Here's how the part is built. I have some questions about the finished solid (model axes, mm). Face numbers are marked on the shaded views. A direction names the side the tool comes from. Round coordinates to 2 decimals unless told otherwise and drop trailing zeros. Write each loop counter-clockwise with the first axis right and the second up, starting at its lowest first coordinate (ties: lowest second). Pieces come first, ordered by that corner, then holes. Notation, with made-up numbers: (2, 39.25) - (27, 39.25) arc R17 cw to (27, 45.25) - close; hole circle Ø2 at (-24, 73.25). An arc over 180 degrees is marked (long way). Use one line per item in the form item = value. Start each with the question number.
1. If I drill on line 1 along Z through (x, y) = (546.45, 0); line 2 along X through (y, z) = (2.25, -6.5); line 3 along Y through (x, z) = (547.5, -6.25), over which ranges is the centre line in solid material (lowest first)?
2. I want a section at B-B, the plane z = 0. State how many separate pieces and enclosed holes the cut face has, plus the area to 3 significant figures.
3. I want a section at A-A, the plane y = 0. List the corners of the cut face in (x, z) for me, plus the area to 3 significant figures.
4. Will these pins go through, and if not, where does the flat tip stop? pin 1 (8 mm diameter, centred on y = 0, z = 0, fed in from -X); pin 2 (6 mm diameter, centred on x = 550, z = 0.5, fed in from +Y); pin 3 (1.5 mm diameter, centred on x = 552.5, z = -5.5, fed in from -Y); pin 4 (3.5 mm diameter, centred on x = 557.15, z = 0, fed in from -Y).
5. I want a section at C-C, the plane z = 8. List the corners of the cut face in (x, y) for me, plus the area to 3 significant figures.
6. Which directions (+Z, -Z, +X, -X, +Y, -Y) give clear straight access to the entire face, cutting with the end or side of a thin tool? Please do the marked faces 4 and 5.
7. I want a section at D-D, the plane y = -6. List the corners of the cut face in (x, z) for me, plus the area to 3 significant figures.
8. We'd pull the mould along Y, two halves only. Please class the marked faces 1, 2 and 3: +Y half, -Y half, draft (parallel to the pull), parting line (faces both ways), or undercut.
```python
from build123d import *

# Parameters (mm, degrees)
CUT_EXTRUDE1_DEPTH      = 561.867355885
CUT_EXTRUDE1_DEPTH_BACK = 561.867355885
SKETCH3_R               = 1.5
SKETCH13_R              = 1
CUT_EXTRUDE2_DEPTH      = 20.974512648


with BuildPart() as part:
    # Sketch2 → Revolve1 (revolve)
    with BuildSketch(Plane.XY, mode=Mode.PRIVATE) as revolve1_sk:
        Polygon((560.650925037, 5), (560.650925037, 7.5), (552.150925037, 7.5), (552.150925037, 6.5), (548.150925037, 6.5), (548.150925037, 7.5), (548.150925037, 11.016604582), (545.650925037, 11.016604582), (545.650925037, 5), align=None)
    revolve(revolve1_sk.sketch.rotate(Axis((542.916757592, 0, 0), (1, 0, 0)), 180), axis=Axis((542.916757592, 0, 0), (1, 0, 0)))

    # Sketch3 → Cut-Extrude1 (cut, two sides: drawn at the far end of the back side and taken through both)
    with BuildSketch(Plane(origin=(0, 0, 0), x_dir=(1, 0, 0), z_dir=(0, 1, 0)).offset(-CUT_EXTRUDE1_DEPTH_BACK)):
        with Locations(Location((557.150925037, 0, 0), (0, 0, 270))):
            Circle(SKETCH3_R)
    extrude(amount=CUT_EXTRUDE1_DEPTH + CUT_EXTRUDE1_DEPTH_BACK, mode=Mode.SUBTRACT)

    # Sketch13 → Cut-Extrude2 (cut, through all)
    with BuildSketch(Plane(origin=(548.150925037, 0, 0), x_dir=(0, 0, -1), z_dir=(1, 0, 0))):
        with Locations(Location((0, 8, 0), (0, 0, 90))):
            Circle(SKETCH13_R)
        with Locations(Location((5.656854249, 5.656854249, 0), (0, 0, 90))):
            Circle(SKETCH13_R)
        with Locations(Location((8, 0, 0), (0, 0, 90))):
            Circle(SKETCH13_R)
        with Locations(Location((5.656854249, -5.656854249, 0), (0, 0, 90))):
            Circle(SKETCH13_R)
        with Locations(Location((0, -8, 0), (0, 0, 90))):
            Circle(SKETCH13_R)
        with Locations(Location((-5.656854249, -5.656854249, 0), (0, 0, 90))):
            Circle(SKETCH13_R)
        with Locations(Location((-8, 0, 0), (0, 0, 90))):
            Circle(SKETCH13_R)
        with Locations(Location((-5.656854249, 5.656854249, 0), (0, 0, 90))):
            Circle(SKETCH13_R)
    extrude(amount=-CUT_EXTRUDE2_DEPTH, mode=Mode.SUBTRACT)


solid = part.part
```
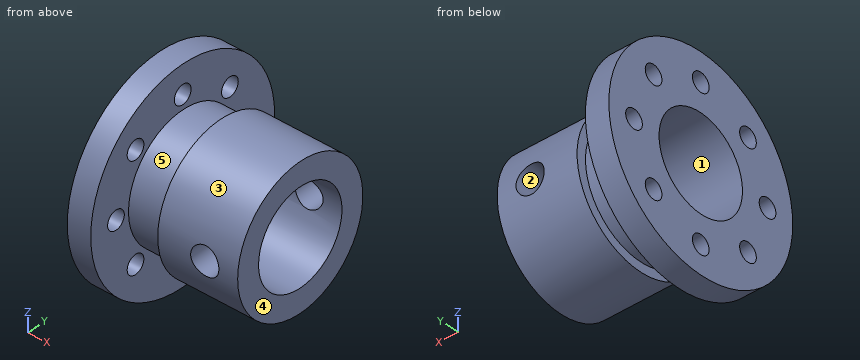
Model answer:
q1.line_1 = -11.02 to -9, -7 to -5, 5 to 7, 9 to 11.02
q1.line_2 = 545.65 to 548.15, 552.15 to 560.65
q1.line_3 = -9.07 to -6.46, -4.85 to 4.85, 6.46 to 9.07
q2.separate_pieces = 6
q2.enclosed_holes = 0
q2.area = 59.6 mm2
q3.outline = (545.65, -11.02) - (548.15, -11.02) - (548.15, -9) - (545.65, -9) - close; (545.65, -7) - (548.15, -7) - (548.15, -6.5) - (552.15, -6.5) - (552.15, -7.5) - (560.65, -7.5) - (560.65, -5) - (545.65, -5) - close; (545.65, 5) - (560.65, 5) - (560.65, 7.5) - (552.15, 7.5) - (552.15, 6.5) - (548.15, 6.5) - (548.15, 7) - (545.65, 7) - close; (545.65, 9) - (548.15, 9) - (548.15, 11.02) - (545.65, 11.02) - close
q3.area = 74.6 mm2
q4.pin_1 = through
q4.pin_2 = 11.02
q4.pin_3 = -5.8
q4.pin_4 = -7.5
q5.outline = (545.65, -7.57) - (548.15, -7.57) - (548.15, -1) - (545.65, -1) - close; (545.65, 1) - (548.15, 1) - (548.15, 7.57) - (545.65, 7.57) - close
q5.area = 32.9 mm2
q6.face_4 = +Z, -Z, +X, +Y, -Y
q6.face_5 = none
q7.outline = (545.65, -9.24) - (548.15, -9.24) - (548.15, -6.6) - (545.65, -6.6) - close; (545.65, -4.72) - (548.15, -4.72) - (548.15, -2.5) - (552.15, -2.5) - (552.15, -4.5) - (560.65, -4.5) - (560.65, 4.5) - (552.15, 4.5) - (552.15, 2.5) - (548.15, 2.5) - (548.15, 4.72) - (545.65, 4.72) - close; (545.65, 6.6) - (548.15, 6.6) - (548.15, 9.24) - (545.65, 9.24) - close; hole circle Ø3 at (557.15, 0)
q7.area = 126 mm2
q8.face_1 = undercut
q8.face_2 = draft
q8.face_3 = parting line
